Here's how the part is built. I have some questions about the finished solid (model axes, mm). A direction names the side the tool comes from. Round coordinates to 2 decimals unless told otherwise and drop trailing zeros. Write each loop counter-clockwise with the first axis right and the second up, starting at its lowest first coordinate (ties: lowest second). Pieces come first, ordered by that corner, then holes. Notation, with made-up numbers: (-26.75, -34.5) - (30.25, -34.5) arc R20 ccw to (30.25, -4.5) - close; hole circle Ø5 at (67, 25.5). An arc over 180 degrees is marked (long way). Return JSON: item names as keys, results as strings. Group by question number.
Autodesk Inventor part; units mm, degrees
sketch "Эскиз1" plane through (0, 0, 0) normal (0, 1, 0) x (-1, 0, 0)
  line L0 (6, 4) -> (-6, 4)
  line L1 (-6, 4) -> (-6, -4)
  line L2 (-6, -4) -> (6, -4)
  line L3 (6, -4) -> (6, 4)
  line L4 (6, 4) -> (-6, -4) construction
  line L5 (-6, 4) -> (6, -4) construction
  point P0 (0, 0)
  dimension "d0" = 12
  dimension "d1" = 8
extrude "Выдавливание1" add sketch "Эскиз1" along normal mid plane 55
sketch "Эскиз2" plane through (-6, 27.5, 4) normal (0, 0, 1) x (1, 0, 0)
  circle A0 centre (6, -13) radius 1.75
  line L0 (0, 0) -> (12, 0)
  line L1 (6, 11) -> (6, -66) construction
  point P0 (6, -27.5)
  dimension "d4" = 13
  dimension "d5" = 3.5
extrude "Выдавливание2" cut sketch "Эскиз2" against normal up to next
sketch "Эскиз3" plane through (-6, 27.5, 4) normal (0, 0, 1) x (1, 0, 0)
  circle A0 centre (6, -13) radius 1.75
  circle A1 centre (6, -13) radius 3
  point P0 (6, -27.5)
  dimension "d8" = 6
extrude "Выдавливание3" cut sketch "Эскиз3" against normal blind 4.5
pattern_linear "Прямоуг.массив1" count 2 spacing 25 along (0, -1, 0) of "Выдавливание3", "Выдавливание2"
properties part number "Направляющая"
1) If we mould it in two halves opening along Y, with no side actions, what happens to faces 3 (the flat face through (-6, 0, 0)), 4 (the flat face through (0, 27.5, 0)), 5 (the cylindrical face through (-0.228, 16.235, -2.226))? For each: released by +Y, released by -Y, zero draft, split by the parting line, or undercut.
2) For faces 1 (the flat face through (0, 0, -4)), 2 (the flat face through (0, 12.5, -0.5)), which set-ups out of +Z, -Z, +X, -X, +Y, -Y let a thin tool reach every point of the face, with its end or its side?
3) Imagine slicing it at A-A (y = 14.5). Please give me the cut outline in (x, z).
4) Will these pins go through, and if not, where does the flat tip stop? pin 1 Ø5 at (x, y) = (0, -10.5) entering from +Z; pin 2 Ø2 at (x, y) = (0, -10.5) entering from -Z.
5) Imagine slicing it at D-D (x = 2.25). Please give me the cut outline in (y, z), plus the area to 3 significant figures.
6) Imagine slicing it at C-C (z = -2). Please give me the cut outline in (x, y).
7) Imagine slicing it at B-B (x = 0). Please give me the cut outline in (y, z), plus the area to 4 significant figures.
8) I need wall thicknesses on line 1 along Y through (x, z) = (0, -3.1); line 2 along Y through (x, z) = (0, 0.5); line 3 along Z through (x, y) = (2, -8.5). Which ranges of each line are inside material? Lowest first, please.
Results found:
{
 "1": {"face 3": "zero draft", "face 4": "released by +Y", "face 5": "undercut"},
 "2": {"face 1": "-Z, +X, -X, +Y, -Y", "face 2": "+Z"},
 "3": {"outline": "(-6, -4) - (-1.75, -4) - (-1.75, -0.5) - (-3, -0.5) - (-3, 4) - (-6, 4) - close; (1.75, -4) - (6, -4) - (6, 4) - (3, 4) - (3, -0.5) - (1.75, -0.5) - close"},
 "4": {"pin 1": "stops at z = -0.5", "pin 2": "passes through"},
 "5": {"outline": "(-27.5, -4) - (27.5, -4) - (27.5, 4) - (16.48, 4) - (16.48, -0.5) - (12.52, -0.5) - (12.52, 4) - (-8.52, 4) - (-8.52, -0.5) - (-12.48, -0.5) - (-12.48, 4) - (-27.5, 4) - close", "area": "404 mm²"},
 "6": {"outline": "(-6, -27.5) - (6, -27.5) - (6, 27.5) - (-6, 27.5) - close; hole circle Ø3.5 at (0, -10.5); hole circle Ø3.5 at (0, 14.5)"},
 "7": {"outline": "(-27.5, -4) - (-12.25, -4) - (-12.25, -0.5) - (-13.5, -0.5) - (-13.5, 4) - (-27.5, 4) - close; (-8.75, -4) - (12.75, -4) - (12.75, -0.5) - (11.5, -0.5) - (11.5, 4) - (-7.5, 4) - (-7.5, -0.5) - (-8.75, -0.5) - close; (16.25, -4) - (27.5, -4) - (27.5, 4) - (17.5, 4) - (17.5, -0.5) - (16.25, -0.5) - close", "area": "361.5 mm²"},
 "8": {"line 1": "y = -27.5 to -12.25, -8.75 to 12.75, 16.25 to 27.5", "line 2": "y = -27.5 to -13.5, -7.5 to 11.5, 17.5 to 27.5", "line 3": "z = -4 to -0.5"}
}
